from build123d import *

# Parameters (mm, degrees)
F0_R         = 7.5
F1_DEPTH     = 35
F2_DEPTH     = 2
F3_SIZE      = 0.5
F4_R         = 5
F5_T1_DEPTH  = 4.6188021535
F5_T3_DEPTH  = 4.6188021535
F5_T5_DEPTH  = 4.6188021535
F5_T7_DEPTH  = 4.6188021535
F5_T9_DEPTH  = 4.6188021535
F5_T11_DEPTH = 4.6188021535
F5_T13_DEPTH = 4.6188021535
F5_T15_DEPTH = 4.6188021535
F5_T17_DEPTH = 4.6188021535
F5_T19_DEPTH = 4.6188021535
F5_T21_DEPTH = 4.6188021535
F5_T23_DEPTH = 4.6188021535
F5_T25_DEPTH = 4.6188021535
F5_T27_DEPTH = 4.6188021535
F5_T29_DEPTH = 4.6188021535
F5_T32_ANGLE = 60
F5_T34_ANGLE = 60
F5_T36_ANGLE = 60
F5_T38_ANGLE = 60
F5_T40_ANGLE = 60
F5_T42_ANGLE = 60
F5_T44_ANGLE = 60
F5_T46_ANGLE = 60
F5_T48_ANGLE = 60
F5_T50_ANGLE = 60
F5_T52_ANGLE = 60
F5_T54_ANGLE = 60
F5_T56_ANGLE = 60
F5_T58_ANGLE = 60
F5_T60_ANGLE = 60
F5_T62_ANGLE = 60
F5_T64_ANGLE = 60
F5_T66_ANGLE = 60


# Not quite as in the source:
# - a fillet or chamfer that OpenCascade refuses, or shapes differently, is made with other operations: its cross-section is extruded or revolved along the edge and cut away or added


with BuildPart() as f1:
    # F0 (on Top) → F1 (new body)
    with BuildSketch(Plane.XY):
        Polygon((-10.3923048454, 18), (-5.1961524227, 9), (5.1961524227, 9), (10.3923048454, 18), (5.1961524227, 27), (-5.1961524227, 27), align=None)
        with Locations((0, 18)):
            Circle(F0_R, mode=Mode.SUBTRACT)
        Polygon((5.1961524227, 9), (-5.1961524227, 9), (-10.3923048454, 0), (-5.1961524227, -9), (5.1961524227, -9), (10.3923048454, 0), align=None)
        Circle(F0_R, mode=Mode.SUBTRACT)
        Polygon((-10.3923048454, 0), (-5.1961524227, 9), (-10.3923048454, 18), (-20.7846096908, 18), (-25.9807621135, 9), (-20.7846096908, 0), align=None)
        with Locations((-15.5884572681, 9)):
            Circle(F0_R, mode=Mode.SUBTRACT)
        Polygon((10.3923048454, 18), (5.1961524227, 9), (10.3923048454, 0), (20.7846096908, 0), (25.9807621135, 9), (20.7846096908, 18), align=None)
        with Locations((15.5884572681, 9)):
            Circle(F0_R, mode=Mode.SUBTRACT)
        Polygon((-5.1961524227, -9), (-10.3923048454, 0), (-20.7846096908, 0), (-25.9807621135, -9), (-20.7846096908, -18), (-10.3923048454, -18), align=None)
        with Locations((-15.5884572681, -9)):
            Circle(F0_R, mode=Mode.SUBTRACT)
        Polygon((20.7846096908, 0), (10.3923048454, 0), (5.1961524227, -9), (10.3923048454, -18), (20.7846096908, -18), (25.9807621135, -9), align=None)
        with Locations((15.5884572681, -9)):
            Circle(F0_R, mode=Mode.SUBTRACT)
        Polygon((5.1961524227, -9), (-5.1961524227, -9), (-10.3923048454, -18), (-5.1961524227, -27), (5.1961524227, -27), (10.3923048454, -18), align=None)
        with Locations((0, -18)):
            Circle(F0_R, mode=Mode.SUBTRACT)
    extrude(amount=F1_DEPTH)

    # F0 (on Top) → F2 (join)
    with BuildSketch(Plane.XY):
        with Locations((-15.5884572681, 9)):
            Circle(F0_R)
        with Locations((-15.5884572681, -9)):
            Circle(F0_R)
        with Locations((0, 18)):
            Circle(F0_R)
        Circle(F0_R)
        with Locations((15.5884572681, 9)):
            Circle(F0_R)
        with Locations((15.5884572681, -9)):
            Circle(F0_R)
        with Locations((0, -18)):
            Circle(F0_R)
    extrude(amount=F2_DEPTH)

    # F3
    f3_edges = [f1.edges().sort_by_distance(p)[0] for p in [
        (-7.5, 18, 35),
        (-23.088457, 9, 35),
        (-7.5, 0, 35),
        (-23.088457, -9, 35),
        (8.088457, 9, 35),
        (8.088457, -9, 35),
        (-7.5, -18, 35),
    ]]
    chamfer(f3_edges, length=F3_SIZE)

    # F4
    f4_edges = [f1.edges().sort_by_distance(p)[0] for p in [
        (-25.980762, 9, 17.5),
        (-20.78461, 18, 17.5),
        (-10.392305, 18, 17.5),
        (-5.196152, 27, 17.5),
        (5.196152, 27, 17.5),
        (10.392305, 18, 17.5),
        (20.78461, 18, 17.5),
        (25.980762, 9, 17.5),
        (20.78461, 0, 17.5),
        (25.980762, -9, 17.5),
        (20.78461, -18, 17.5),
        (10.392305, -18, 17.5),
        (5.196152, -27, 17.5),
        (-5.196152, -27, 17.5),
        (-10.392305, -18, 17.5),
        (-20.78461, -18, 17.5),
        (-25.980762, -9, 17.5),
        (-20.78461, 0, 17.5),
    ]]
    fillet(f4_edges, radius=F4_R)

    # F5: chamfer of 1.5 x 2.5980762114 on 36 edges, made by hand

    # F5_s2 → F5_t1 (cut)
    with BuildSketch(Plane.YZ.offset(13.2790561914)):
        Polygon((-18, 2.5980762114), (-16.5, 0), (-18, 0), align=None)
        Polygon((18, 2.5980762114), (16.5, 0), (18, 0), align=None)
    extrude(amount=F5_T1_DEPTH, mode=Mode.SUBTRACT)

    # F5_s4 → F5_t3 (cut)
    with BuildSketch(Plane(origin=(-8.9489291724, -15.5, 0), x_dir=(0, 0, 1), z_dir=(0.5, 0.8660254038, 0))):
        Polygon((2.5980762114, 18), (0, 16.5), (0, 18), align=None)
    extrude(amount=F5_T3_DEPTH, mode=Mode.SUBTRACT)

    # F5_s6 → F5_t5 (cut)
    with BuildSketch(Plane(origin=(-1.1547005384, -2, 0), x_dir=(0, 0, 1), z_dir=(0.5, 0.8660254038, 0))):
        Polygon((2.5980762114, 27), (0, 25.5), (0, 27), align=None)
    extrude(amount=F5_T5_DEPTH, mode=Mode.SUBTRACT)

    # F5_s8 → F5_t7 (cut)
    with BuildSketch(Plane.YZ.offset(-2.3094010768)):
        Polygon((-27, 2.5980762114), (-25.5, 0), (-27, 0), align=None)
        Polygon((27, 2.5980762114), (25.5, 0), (27, 0), align=None)
    extrude(amount=F5_T7_DEPTH, mode=Mode.SUBTRACT)

    # F5_s10 → F5_t9 (cut)
    with BuildSketch(Plane(origin=(8.9489291724, -15.5, 0), x_dir=(0, 0, 1), z_dir=(-0.5, 0.8660254038, 0))):
        Polygon((2.5980762114, 18), (0, 16.5), (0, 18), align=None)
    extrude(amount=F5_T9_DEPTH, mode=Mode.SUBTRACT)

    # F5_s12 → F5_t11 (cut)
    with BuildSketch(Plane(origin=(6.6395280957, -11.5, 0), x_dir=(0, 0, 1), z_dir=(0.5, -0.8660254038, 0))):
        Polygon((2.5980762114, 18), (0, 16.5), (0, 18), align=None)
    extrude(amount=F5_T11_DEPTH, mode=Mode.SUBTRACT)

    # F5_s14 → F5_t13 (cut)
    with BuildSketch(Plane(origin=(6.6395280957, 11.5, 0), x_dir=(0, 0, 1), z_dir=(0.5, 0.8660254038, 0))):
        Polygon((2.5980762114, 18), (0, 16.5), (0, 18), align=None)
    extrude(amount=F5_T13_DEPTH, mode=Mode.SUBTRACT)

    # F5_s16 → F5_t15 (cut)
    with BuildSketch(Plane.YZ.offset(-17.8978583449)):
        Polygon((-18, 2.5980762114), (-16.5, 0), (-18, 0), align=None)
        Polygon((18, 2.5980762114), (16.5, 0), (18, 0), align=None)
    extrude(amount=F5_T15_DEPTH, mode=Mode.SUBTRACT)

    # F5_s18 → F5_t17 (cut)
    with BuildSketch(Plane(origin=(1.1547005384, -2, 0), x_dir=(0, 0, 1), z_dir=(-0.5, 0.8660254038, 0))):
        Polygon((2.5980762114, 27), (0, 25.5), (0, 27), align=None)
    extrude(amount=F5_T17_DEPTH, mode=Mode.SUBTRACT)

    # F5_s20 → F5_t19 (cut)
    with BuildSketch(Plane(origin=(-1.1547005384, 2, 0), x_dir=(0, 0, 1), z_dir=(0.5, -0.8660254038, 0))):
        Polygon((2.5980762114, 27), (0, 25.5), (0, 27), align=None)
    extrude(amount=F5_T19_DEPTH, mode=Mode.SUBTRACT)

    # F5_s22 → F5_t21 (cut)
    with BuildSketch(Plane(origin=(-6.6395280957, -11.5, 0), x_dir=(0, 0, 1), z_dir=(-0.5, -0.8660254038, 0))):
        Polygon((2.5980762114, 18), (0, 16.5), (0, 18), align=None)
    extrude(amount=F5_T21_DEPTH, mode=Mode.SUBTRACT)

    # F5_s24 → F5_t23 (cut)
    with BuildSketch(Plane(origin=(-6.6395280957, 11.5, 0), x_dir=(0, 0, 1), z_dir=(-0.5, 0.8660254038, 0))):
        Polygon((2.5980762114, 18), (0, 16.5), (0, 18), align=None)
    extrude(amount=F5_T23_DEPTH, mode=Mode.SUBTRACT)

    # F5_s26 → F5_t25 (cut)
    with BuildSketch(Plane(origin=(-8.9489291724, 15.5, 0), x_dir=(0, 0, 1), z_dir=(0.5, -0.8660254038, 0))):
        Polygon((2.5980762114, 18), (0, 16.5), (0, 18), align=None)
    extrude(amount=F5_T25_DEPTH, mode=Mode.SUBTRACT)

    # F5_s28 → F5_t27 (cut)
    with BuildSketch(Plane(origin=(1.1547005384, 2, 0), x_dir=(0, 0, 1), z_dir=(-0.5, -0.8660254038, 0))):
        Polygon((2.5980762114, 27), (0, 25.5), (0, 27), align=None)
    extrude(amount=F5_T27_DEPTH, mode=Mode.SUBTRACT)

    # F5_s30 → F5_t29 (cut)
    with BuildSketch(Plane(origin=(8.9489291724, 15.5, 0), x_dir=(0, 0, 1), z_dir=(-0.5, -0.8660254038, 0))):
        Polygon((2.5980762114, 18), (0, 16.5), (0, 18), align=None)
    extrude(amount=F5_T29_DEPTH, mode=Mode.SUBTRACT)

    # F5_s31 → F5_t32 (revolve, cut)
    with BuildSketch(Plane.YZ.offset(13.2790561914)):
        Polygon((-18, 2.5980762114), (-16.5, 0), (-18, 0), align=None)
    revolve(axis=Axis((13.2790561914, -23, 0), (0, 0, 1)), revolution_arc=F5_T32_ANGLE, mode=Mode.SUBTRACT)

    # F5_s33 → F5_t34 (revolve, cut)
    with BuildSketch(Plane.YZ.offset(17.8978583449)):
        Polygon((-18, 2.5980762114), (-16.5, 0), (-18, 0), align=None)
    revolve(axis=Axis((17.8978583449, -13, 0), (0, 0, 1)), revolution_arc=F5_T34_ANGLE, mode=Mode.SUBTRACT)

    # F5_s35 → F5_t36 (revolve, cut)
    with BuildSketch(Plane.YZ.offset(2.3094010768)):
        Polygon((-27, 2.5980762114), (-25.5, 0), (-27, 0), align=None)
    revolve(axis=Axis((2.3094010768, -22, 0), (0, 0, 1)), revolution_arc=F5_T36_ANGLE, mode=Mode.SUBTRACT)

    # F5_s37 → F5_t38 (revolve, cut)
    with BuildSketch(Plane(origin=(1.1547005384, 2, 0), x_dir=(0, 0, 1), z_dir=(-0.5, -0.8660254038, 0))):
        Polygon((2.5980762114, -27), (0, -25.5), (0, -27), align=None)
    revolve(axis=Axis((20.2072594216, -9, 0), (0, 0, 1)), revolution_arc=F5_T38_ANGLE, mode=Mode.SUBTRACT)

    # F5_s39 → F5_t40 (revolve, cut)
    with BuildSketch(Plane(origin=(8.9489291724, -15.5, 0), x_dir=(0, 0, 1), z_dir=(-0.5, 0.8660254038, 0))):
        Polygon((2.5980762114, -18), (0, -16.5), (0, -18), align=None)
    revolve(axis=Axis((-2.3094010768, -22, 0), (0, 0, 1)), revolution_arc=F5_T40_ANGLE, mode=Mode.SUBTRACT)

    # F5_s41 → F5_t42 (revolve, cut)
    with BuildSketch(Plane(origin=(6.6395280957, -11.5, 0), x_dir=(0, 0, 1), z_dir=(0.5, -0.8660254038, 0))):
        Polygon((2.5980762114, -18), (0, -16.5), (0, -18), align=None)
    revolve(axis=Axis((26.5581123827, 0, 0), (0, 0, -1)), revolution_arc=F5_T42_ANGLE, mode=Mode.SUBTRACT)

    # F5_s43 → F5_t44 (revolve, cut)
    with BuildSketch(Plane.YZ.offset(-13.2790561914)):
        Polygon((-18, 2.5980762114), (-16.5, 0), (-18, 0), align=None)
    revolve(axis=Axis((-13.2790561914, -23, 0), (0, 0, -1)), revolution_arc=F5_T44_ANGLE, mode=Mode.SUBTRACT)

    # F5_s45 → F5_t46 (revolve, cut)
    with BuildSketch(Plane(origin=(8.9489291724, 15.5, 0), x_dir=(0, 0, 1), z_dir=(-0.5, -0.8660254038, 0))):
        Polygon((2.5980762114, -18), (0, -16.5), (0, -18), align=None)
    revolve(axis=Axis((20.2072594216, 9, 0), (0, 0, 1)), revolution_arc=F5_T46_ANGLE, mode=Mode.SUBTRACT)

    # F5_s47 → F5_t48 (revolve, cut)
    with BuildSketch(Plane(origin=(1.1547005384, -2, 0), x_dir=(0, 0, 1), z_dir=(-0.5, 0.8660254038, 0))):
        Polygon((2.5980762114, -27), (0, -25.5), (0, -27), align=None)
    revolve(axis=Axis((-17.8978583449, -13, 0), (0, 0, 1)), revolution_arc=F5_T48_ANGLE, mode=Mode.SUBTRACT)

    # F5_s49 → F5_t50 (revolve, cut)
    with BuildSketch(Plane(origin=(-1.1547005384, 2, 0), x_dir=(0, 0, 1), z_dir=(0.5, -0.8660254038, 0))):
        Polygon((2.5980762114, -27), (0, -25.5), (0, -27), align=None)
    revolve(axis=Axis((17.8978583449, 13, 0), (0, 0, 1)), revolution_arc=F5_T50_ANGLE, mode=Mode.SUBTRACT)

    # F5_s51 → F5_t52 (revolve, cut)
    with BuildSketch(Plane(origin=(-8.9489291724, -15.5, 0), x_dir=(0, 0, 1), z_dir=(0.5, 0.8660254038, 0))):
        Polygon((2.5980762114, -18), (0, -16.5), (0, -18), align=None)
    revolve(axis=Axis((-20.2072594216, -9, 0), (0, 0, 1)), revolution_arc=F5_T52_ANGLE, mode=Mode.SUBTRACT)

    # F5_s53 → F5_t54 (revolve, cut)
    with BuildSketch(Plane.YZ.offset(13.2790561914)):
        Polygon((18, 2.5980762114), (16.5, 0), (18, 0), align=None)
    revolve(axis=Axis((13.2790561914, 23, 0), (0, 0, -1)), revolution_arc=F5_T54_ANGLE, mode=Mode.SUBTRACT)

    # F5_s55 → F5_t56 (revolve, cut)
    with BuildSketch(Plane(origin=(-6.6395280957, 11.5, 0), x_dir=(0, 0, 1), z_dir=(-0.5, 0.8660254038, 0))):
        Polygon((2.5980762114, -18), (0, -16.5), (0, -18), align=None)
    revolve(axis=Axis((-26.5581123827, 0, 0), (0, 0, -1)), revolution_arc=F5_T56_ANGLE, mode=Mode.SUBTRACT)

    # F5_s57 → F5_t58 (revolve, cut)
    with BuildSketch(Plane(origin=(-8.9489291724, 15.5, 0), x_dir=(0, 0, 1), z_dir=(0.5, -0.8660254038, 0))):
        Polygon((2.5980762114, -18), (0, -16.5), (0, -18), align=None)
    revolve(axis=Axis((2.3094010768, 22, 0), (0, 0, 1)), revolution_arc=F5_T58_ANGLE, mode=Mode.SUBTRACT)

    # F5_s59 → F5_t60 (revolve, cut)
    with BuildSketch(Plane(origin=(-1.1547005384, -2, 0), x_dir=(0, 0, 1), z_dir=(0.5, 0.8660254038, 0))):
        Polygon((2.5980762114, -27), (0, -25.5), (0, -27), align=None)
    revolve(axis=Axis((-20.2072594216, 9, 0), (0, 0, 1)), revolution_arc=F5_T60_ANGLE, mode=Mode.SUBTRACT)

    # F5_s61 → F5_t62 (revolve, cut)
    with BuildSketch(Plane.YZ.offset(-2.3094010768)):
        Polygon((27, 2.5980762114), (25.5, 0), (27, 0), align=None)
    revolve(axis=Axis((-2.3094010768, 22, 0), (0, 0, 1)), revolution_arc=F5_T62_ANGLE, mode=Mode.SUBTRACT)

    # F5_s63 → F5_t64 (revolve, cut)
    with BuildSketch(Plane.YZ.offset(-17.8978583449)):
        Polygon((18, 2.5980762114), (16.5, 0), (18, 0), align=None)
    revolve(axis=Axis((-17.8978583449, 13, 0), (0, 0, 1)), revolution_arc=F5_T64_ANGLE, mode=Mode.SUBTRACT)

    # F5_s65 → F5_t66 (revolve, cut)
    with BuildSketch(Plane(origin=(6.6395280957, 11.5, 0), x_dir=(0, 0, 1), z_dir=(0.5, 0.8660254038, 0))):
        Polygon((2.5980762114, -18), (0, -16.5), (0, -18), align=None)
    revolve(axis=Axis((-13.2790561914, 23, 0), (0, 0, -1)), revolution_arc=F5_T66_ANGLE, mode=Mode.SUBTRACT)


solid = f1.part
Work out the finished part from the listing and answer in its coordinate system (mm). A direction names the side the tool comes from. Give positions to 0.01 mm unless a question says otherwise; leave off trailing zeros. Order: outer loops, then holes, each group sorted by start corner. A loop starts at its lowest first (then second) coordinate and runs counter-clockwise, first axis right, second up. Notation, with made-up numbers: (16, 43.25) -> (53, 43.25) arc R21 ccw to (53, 62.25) -> close; hole circle Ø8 at (-11.75, 87). An arc over 180 degrees is marked (long way). One line per item, written item: value.
Item 1: Find section A-A, the plane y = 0. Give the vertices of the cut face in (x, z), plus the area to 3 significant figures.
Answer sheet:
outline: (-21.56, 2.6) -> (-20.06, 0) -> (20.06, 0) -> (21.56, 2.6) -> (21.56, 35) -> (8, 35) -> (7.5, 34.5) -> (7.5, 2) -> (-7.5, 2) -> (-7.5, 34.5) -> (-8, 35) -> (-21.56, 35) -> close
area: 1,010 mm²
Item 2: Straight lines are drawn through the part: probe 1 along Y at (x, z) = (0, 27); probe 2 along Y at (x, z) = (2, 24); probe 3 along X at (y, z) = (-6, 11). For each, find the intervals that lie inside material, in ascending order.
Answer sheet:
probe 1: -27 to -25.5, -10.5 to -7.5, 7.5 to 10.5, 25.5 to 27
probe 2: -27 to -25.23, -10.77 to -7.23, 7.23 to 10.77, 25.23 to 27
probe 3: -24.25 to -22.46, -8.71 to -4.5, 4.5 to 8.71, 22.46 to 24.25
Item 3: A tool of negligible diameter and unlimited length cuts with its end or side. For faces 1 (the flat face through (23.4, -4.53, 18.57)), 2 (the flat face through (15.56, -17.26, 1.32)), 3 (the flat face through (-16, 9, 2)), 4 (the flat face through (-23.4, 4.53, 18.57)), from which of +Z, -Z, +X, -X, +Y, -Y can it reach the whole face along a straight path? Write none if from no direction.
Answer sheet:
face 1: +Z, -Z, +X
face 2: -Z, +X, -Y
face 3: +Z
face 4: +Z, -Z, -X
Item 4: Flat-ended cylindrical pins translate along their axes: P1, Ø3.5, axis at x = 16.5, z = 14.5, coming from the +Y side; P2, Ø1.5, axis at x = -13, y = 13.5, coming from the +Z side; P3, Ø2, axis at y = 11.5, z = 13.5, coming from the +X side. Find the tip coordinate at first contact, or state that the pin passes through.
Answer sheet:
P1: y = 18
P2: z = 2
P3: x = 24.98
Item 5: Determine the mould class of faces 5 (the flat face through (16, 18, 19)), 6 (the conical face through (-20.04, -16.66, 1.28)), 7 (the flat face through (23.367, 4.472, 18.572)) for opening direction Y: released by +Y, released by -Y, zero draft, split by the parting line, or undercut.
Answer sheet:
face 5: released by +Y
face 6: released by -Y
face 7: undercut
Item 6: Find section B-B, the plane z = 5. State how many separate pieces and enclosed holes the cut face has, plus the area to 3 significant figures.
Answer sheet:
separate pieces: 1
enclosed holes: 7
area: 719 mm²
